Here's how the part is built. I have some questions about the finished solid (model axes, mm). A direction names the side the tool comes from. Coordinates: 2 decimals unless noted, no trailing zeros. Loops run counter-clockwise (first coordinate to the right, second up) from the corner with the lowest first, then second, coordinate; pieces in that order, holes last. Notation, with made-up numbers: (15, 68.25) -> (71, 68.25) arc R23 cw to (71, 100.25) -> close; hole circle Ø11 at (43, 43). An arc over 180 degrees is marked (long way). Answer as a JSON object with one key per item and string values. Group by question number.
Q1. I want a section at A-A on y = 15.5. Write out the boundary of the cut face in (x, z).
Q2. I want a section at C-C on x = 28.5. Write out the boundary of the cut face in (y, z), then the cut area to 3 significant figures.
Q3. I'm going to push flat-ended pins straight in: pin 1 (14.5 mm diameter, centred on x = -20, y = -7, fed in from +Z); pin 2 (1.5 mm diameter, centred on y = 14.5, z = 82, fed in from -X); pin 3 (8 mm diameter, centred on x = 6, y = -5, fed in from -Z); pin 4 (3 mm diameter, centred on x = 52.5, z = 111, fed in from -Y). Where does each tip first touch, or does it pass through?
Q4. On a 3-axis mill with a long thin cutter (end or side, diameter ignored), from which of +Z, -Z, +X, -X, +Y, -Y can I reach the whole of each face in a straight line? I mean faces 5 (the cylindrical face through (44.5, -5.85, -7.4)), 6 (the cylindrical face through (34.07, 22.85, 133.71)), 7 (the cylindrical face through (52.48, 31.97, 121.92)), 8 (the flat face through (-1, -16, 0)). Say none if no direction works.
Q5. Thinking about a two-plate mould opening in Z: for faces 1 (the flat face through (15, 18, 40)), 2 (the flat face through (72.5, 20, 21)), 3 (the flat face through (-33.46, 23.92, 50.7)), 4 (the cylindrical face through (26.707, 17.325, 110.814)), which applies, released by +Z, released by -Z, zero draft, split by the parting line, or undercut?
Q6. I want a section at D-D on z = 107. Write out the boundary of the cut face in (x, y).
Q7. I want a section at B-B on y = -6. Write out the boundary of the cut face in (x, z), then the cut area to 3 significant figures.
Q8. I need wall thicknesses on line 1 (Z direction, x = 38.5, y = 14.5); line 2 (Z direction, x = 38.5, y = 23.25); line 3 (Y direction, x = -9, z = -8). Which ranges of each line are inside material? Lowest first, please.
```python
from build123d import *

# Parameters (mm, degrees)
F0_W     = 145
F0_H     = 60
F1_DEPTH = 15
F3_START = -18
F3_DEPTH = 12
F4_START = -12
F2_R     = 26
F4_DEPTH = 22
F5_START = -5
F2_R_2   = 16
F5_DEPTH = 25


with BuildPart() as f1:
    # F0 (on Top) → F1 (new body)
    with BuildSketch(Plane.XY):
        Rectangle(F0_W, F0_H)
        with BuildLine():
            ThreePointArc((-37.5, -13), (-44.5, -6), (-37.5, 1))
            Line((-37.5, 1), (37.5, 1))
            ThreePointArc((37.5, 1), (44.5, -6), (37.5, -13))
            Line((37.5, -13), (-37.5, -13))
        make_face(mode=Mode.SUBTRACT)
    extrude(amount=-F1_DEPTH)

    # F2 (on Front) → F3 (join)
    with BuildSketch(Plane.XZ.offset(F3_START)):
        with BuildLine():
            Line((72.5, 0), (72.5, 100))
            ThreePointArc((72.5, 100), (38.5, 66), (4.5, 100))
            Line((4.5, 100), (-72.5, 0))
            Line((-72.5, 0), (-63.7343847897, 0))
            Line((-63.7343847897, 0), (65.0060102344, 0))
            Line((65.0060102344, 0), (72.5, 0))
        make_face()
    extrude(amount=-F3_DEPTH)

    # F2 (on Front) → F4 (join)
    with BuildSketch(Plane.XZ.offset(F4_START)):
        with BuildLine():
            ThreePointArc((4.5, 100), (38.5, 66), (72.5, 100))
            ThreePointArc((72.5, 100), (38.5, 134), (4.5, 100))
        make_face()
        with Locations((38.5, 100)):
            Circle(F2_R, mode=Mode.SUBTRACT)
    extrude(amount=-F4_DEPTH)

    # F2 (on Front) → F5 (join)
    with BuildSketch(Plane.XZ.offset(F5_START)):
        with Locations((38.5, 100)):
            Circle(F2_R)
        with Locations((38.5, 100)):
            Circle(F2_R_2, mode=Mode.SUBTRACT)
    extrude(amount=-F5_DEPTH)


solid = f1.part
```
Result set:
{
 "1": {"outline": "(-72.5, -15) -> (72.5, -15) -> (72.5, 0) -> (-72.5, 0) -> close; circle Ø68 at (38.5, 100); hole circle Ø32 at (38.5, 100)"},
 "2": {"outline": "(-30, -15) -> (-13, -15) -> (-13, 0) -> (-30, 0) -> close; (1, -15) -> (30, -15) -> (30, 67.5) -> (34, 67.5) -> (34, 76) -> (30, 76) -> (30, 87.51) -> (5, 87.51) -> (5, 76) -> (12, 76) -> (12, 67.5) -> (18, 67.5) -> (18, 0) -> (1, 0) -> close; (5, 112.49) -> (30, 112.49) -> (30, 124) -> (34, 124) -> (34, 132.5) -> (12, 132.5) -> (12, 124) -> (5, 124) -> close", "area": "2,450 mm²"},
 "3": {"pin 1": "stops at z = 0", "pin 2": "stops at x = 9.2", "pin 3": "passes through", "pin 4": "stops at y = 5"},
 "4": {"face 5": "+Z, -Z", "face 6": "none", "face 7": "+Y", "face 8": "+X, -X, -Y"},
 "5": {"face 1": "undercut", "face 2": "zero draft", "face 3": "released by +Z", "face 4": "undercut"},
 "6": {"outline": "(5.23, 12) -> (13.46, 12) -> (13.46, 5) -> (24.11, 5) -> (24.11, 30) -> (13.46, 30) -> (13.46, 34) -> (5.23, 34) -> close; (52.89, 5) -> (63.54, 5) -> (63.54, 12) -> (71.77, 12) -> (71.77, 34) -> (63.54, 34) -> (63.54, 30) -> (52.89, 30) -> close"},
 "7": {"outline": "(-72.5, -15) -> (-44.5, -15) -> (-44.5, 0) -> (-72.5, 0) -> close; (44.5, -15) -> (72.5, -15) -> (72.5, 0) -> (44.5, 0) -> close", "area": "840 mm²"},
 "8": {"line 1": "z = -15 to 0, 66 to 84, 116 to 134", "line 2": "z = -15 to 84, 116 to 134", "line 3": "y = -30 to -13, 1 to 30"}
}
